from build123d import *

# Parameters (mm, degrees)
SKETCH1_R           = 1.6
BOSS_EXTRUDE1_DEPTH = 0.4


with BuildPart() as part:
    # Sketch1 → Boss-Extrude1 (new body)
    with BuildSketch(Plane(origin=(0, 0, 0), x_dir=(1, 0, 0), z_dir=(0, 1, 0))):
        with BuildLine():
            Line((29.237843605, 13.960963482), (24.049079653, -21.711788683))
            ThreePointArc((24.049079653, -21.711788683), (17.208573183, -27.452231403), (9.060814288, -31.107260317))
            Line((9.060814288, -31.107260317), (-9.060814288, -31.107260317))
            ThreePointArc((-9.060814288, -31.107260317), (-24.689356555, 20.980840614), (29.237843605, 13.960963482))
        make_face()
        with Locations(Location((-17.5, 23, 0), (0, 0, 270))):
            Circle(SKETCH1_R, mode=Mode.SUBTRACT)
        with Locations(Location((-17.5, -23, 0), (0, 0, 270))):
            Circle(SKETCH1_R, mode=Mode.SUBTRACT)
        with Locations(Location((17.5, -23, 0), (0, 0, 270))):
            Circle(SKETCH1_R, mode=Mode.SUBTRACT)
        with Locations(Location((17.5, 23, 0), (0, 0, 270))):
            Circle(SKETCH1_R, mode=Mode.SUBTRACT)
        with BuildLine():
            Line((-4, -24.107260317), (4, -24.107260317))
            ThreePointArc((4, -24.107260317), (8.793181532, -28.027829543), (11.685431528, -22.552398764))
            ThreePointArc((11.685431528, -22.552398764), (0, 25.4), (-11.685431528, -22.552398764))
            ThreePointArc((-11.685431528, -22.552398764), (-8.793181532, -28.027829543), (-4, -24.107260317))
        make_face(mode=Mode.SUBTRACT)
    extrude(amount=BOSS_EXTRUDE1_DEPTH)


solid = part.part
Could you check a few things on this model? Use its own coordinates, in mm. Coordinates: 2 decimals unless noted, no trailing zeros. Loops run counter-clockwise (first coordinate to the right, second up) from the corner with the lowest first, then second, coordinate; pieces in that order, holes last. Notation, with made-up numbers: (52, 88.5) -> (95, 88.5) arc R21 ccw to (95, 116.5) -> close; hole circle Ø4 at (13, 64). An arc over 180 degrees is marked (long way). Answer in a Markdown table with one row per item.
(1) Imagine slicing it at A-A (x = 0). List the corners of the cut face in (y, z) for me.
Results found:
| item | result |
|---|---|
| outline | (0, -32.4) -> (0.4, -32.4) -> (0.4, -25.4) -> (0, -25.4) -> close; (0, 24.11) -> (0.4, 24.11) -> (0.4, 31.11) -> (0, 31.11) -> close |
(2) Imagine slicing it at B-B (z = 16). List the corners of the cut face in (x, y) for me, plus the area to 3 significant figures.
Results found:
| item | result |
|---|---|
| outline | (-28.17, 0) -> (-19.73, 0) -> (-19.73, 0.4) -> (-28.17, 0.4) -> close; (19.73, 0) -> (24.88, 0) -> (24.88, 0.4) -> (19.73, 0.4) -> close |
| area | 5.44 mm^2 |
(3) If I drill on probe 1 along X at (y, z) = (0.25, 23); probe 2 along Z at (x, y) = (0.5, 0.35); probe 3 along X at (y, z) = (0.35, -16), over which ranges is the centre line in solid material (lowest first)?
Results found:
| item | result |
|---|---|
| probe 1 | x = -22.82 to -19.1, -15.9 to -11.84, 11.84 to 15.9, 19.1 to 22.82 |
| probe 2 | z = -32.4 to -25.4, 24.11 to 31.11 |
| probe 3 | x = -28.17 to -19.73, 19.73 to 28.17 |
(4) Will this pin go through, and if not, where does the flat tip stop? pin 1 Ø13 at (x, z) = (8, 24.11) entering from +Y.
Results found:
| item | result |
|---|---|
| pin 1 | stops at y = 0.4 |
(5) Imagine slicing it at D-D (z = -23). List the corners of the cut face in (x, y) for me, plus the area to 3 significant figures.
Results found:
| item | result |
|---|---|
| outline | (-22.82, 0) -> (-19.1, 0) -> (-19.1, 0.4) -> (-22.82, 0.4) -> close; (-15.9, 0) -> (-10.78, 0) -> (-10.78, 0.4) -> (-15.9, 0.4) -> close; (10.78, 0) -> (15.9, 0) -> (15.9, 0.4) -> (10.78, 0.4) -> close; (19.1, 0) -> (22.82, 0) -> (22.82, 0.4) -> (19.1, 0.4) -> close |
| area | 7.07 mm^2 |
(6) Thinking about a two-plate mould opening in Z: for faces 1 (the face through (0.947, 0.197, -25.382)), 2 (the face through (-24, 0, -10)), 3 (the face through (17.31, 0.2, 27.39)), which applies, released by +Z, released by -Z, zero draft, split by the parting line, or undercut?
Results found:
| item | result |
|---|---|
| face 1 | undercut |
| face 2 | zero draft |
| face 3 | released by +Z |
(7) Imagine slicing it at C-C (y = 0.2). List the corners of the cut face in (x, z) for me, plus the area to 3 significant figures.
Results found:
| item | result |
|---|---|
| outline | (-9.06, 31.11) arc R32.4 ccw (long way) to (29.24, -13.96) -> (24.05, 21.71) arc R32.4 ccw to (9.06, 31.11) -> close; hole circle Ø3.2 at (-17.5, -23); hole circle Ø3.2 at (-17.5, 23); hole (-11.69, 22.55) arc R25.4 ccw (long way) to (11.69, 22.55) arc R4 ccw (long way) to (4, 24.11) -> (-4, 24.11) arc R4 ccw (long way) to start; hole circle Ø3.2 at (17.5, -23); hole circle Ø3.2 at (17.5, 23) |
| area | 1,050 mm^2 |
